Autodesk Inventor part; units mm, degrees
ref_plane "YZ Plane" through (0, 0, 0) normal (1, 0, 0) x (0, 1, 0)
ref_plane "XZ Plane" through (0, 0, 0) normal (0, 1, 0) x (-1, 0, 0)
ref_plane "XY Plane" through (0, 0, 0) normal (0, 0, 1) x (1, 0, 0)
sketch "スケッチ1" plane through (0, 0, 0) normal (0, 0, 1) x (1, 0, 0)
  circle A0 centre (0, 0) radius 2.25
  dimension "d0" = 4.5
extrude "押し出し1" add sketch "スケッチ1" along normal blind 2.5
sketch "スケッチ2" plane through (0, 0, 0) normal (0, 0, -1) x (-1, 0, 0)
  circle A0 centre (0, 0) radius 1.25
  dimension "d3" = 2.5
extrude "押し出し2" add sketch "スケッチ2" along normal blind 4
chamfer "面取り1" distance 0.1 angle 45 1 edges at (-2.25, 0, 2.5)
thread "ねじ1"
properties part number "M2.5×4" material "ステンレス鋼"
Read the model definition and answer for the solid it produces. Units are mm, in the model's axes. A direction names the side the tool comes from. Coordinates: 2 decimals unless noted, no trailing zeros. Order: outer loops, then holes, each group sorted by start corner. A loop starts at its lowest first (then second) coordinate and runs counter-clockwise, first axis right, second up. Notation, with made-up numbers: M 8,87 L 18,87 A9 ccw 18,99 Z; hole C 0.25,5.5 d10. An arc over 180 degrees is marked long. Put each result on its own line as item: value. Start each with the question number.
Item 1: For faces 1 (the face through (0.27, 1.22, -1.97)), 2 (the face through (-0.29, -2.23, 1.18)), determine the directions among +Z, -Z, +X, -X, +Y, -Y from which every point of the face is accessible in a straight line to the end or side of a thin tool.
Item 2: Section D-D, the plane z = 0.5 is taken. Determine the outline of the cut face in (x, y).
Item 3: Section C-C, the plane z = -1 is taken. Determine the outline of the cut face in (x, y).
Item 4: Given pin 1 Ø2 at (x, z) = (0.5, -3) entering from -Y, flat-ended and moving along its own axis, determine where the tip first touches the part or whether it passes through.
Item 5: Consider probe 1 along Z at (x, y) = (1.1, 1.3); probe 2 along X at (y, z) = (-1.35, 2.25); probe 3 along X at (y, z) = (0.75, 1). Determine where each line is inside the solid, lowest interval first. Write a range as [from, to].
Item 6: Section A-A, the plane x = 0 is taken. Determine the outline of the cut face in (y, z).
Computed:
1. face 1: -Z
1. face 2: +Z, -Z
2. outline: C 0,0 d4.5
3. outline: C 0,0 d2.5
4. pin 1: stops at y = -1.25
5. probe 1: z = [0, 2.5]
5. probe 2: x = [-1.8, 1.8]
5. probe 3: x = [-2.12, 2.12]
6. outline: M -2.25,0 L -1.25,0 L -1.25,-4 L 1.25,-4 L 1.25,0 L 2.25,0 L 2.25,2.4 L 2.15,2.5 L -2.15,2.5 L -2.25,2.4 Z
